The listing builds one solid part. Answer for the finished solid, in the listing's coordinates (mm). A direction names the side the tool comes from. Give positions to 0.01 mm unless a question says otherwise; leave off trailing zeros. Order: outer loops, then holes, each group sorted by start corner. A loop starts at its lowest first (then second) coordinate and runs counter-clockwise, first axis right, second up. Notation, with made-up numbers: (78.25, -32) - (100.25, -32) arc R10 cw to (100.25, -15) - close; hole circle Ø6 at (-38.5, 83). An arc over 180 degrees is marked (long way). Answer as a JSON object with one key per item and string values. Group by question number.
Q1. A cutting plane is placed at A-A, the plane y = 21. Give the vertices of the cut face in (x, z).
Q2. A cutting plane is placed at C-C, the plane y = 12. Give the vertices of the cut face in (x, z).
Q3. A cutting plane is placed at B-B, the plane z = 3.55. Count the separate pieces of the cut face and the enclosed holes in it, and give its area (3 significant figures).
Q4. The mould has two halves that part along X. Classify faces 4 (the face through (-1, 0, 6)), 5 (the face through (70.85, 0, 4)), 6 (the face through (76.592, -21.601, 1.268)): released by +X, released by -X, zero draft, split by the parting line, or undercut.
Q5. Given pin 1 (5 mm diameter, centred on x = 78.5, y = -21, fed in from +Z); pin 2 (1.8 mm diameter, centred on x = 23.5, y = -15, fed in from -Z), each flat-ended and moving along its own axis, determine where each tip first touches the part or whether it passes through.
Q6. Consider line 1 (Y direction, x = 0, z = 2.25) (3 decimals); line 2 (Z direction, x = 71, y = 4.5); line 3 (X direction, y = -0.5, z = 5.05). Determine where each line is inside the solid, lowest interval first.
Q7. For faces 1 (the face through (-79, 0, 2.5)), 2 (the face through (78, 0, 2.5)), 3 (the face through (80.408, 21.601, 1.268)), determine the directions among +Z, -Z, +X, -X, +Y, -Y from which every point of the face is accessible in a straight line to the end or side of a thin tool.
from build123d import *

# Parameters (mm, degrees)
ESQUISSE1_W             = 172
ESQUISSE1_H             = 55
BOSS_EXTRU_1_DEPTH      = 6
ESQUISSE2_W             = 15.15
ESQUISSE2_H             = 55
ENL_V_MAT_EXTRU_1_DEPTH = 3.5
ESQUISSE3_R             = 2
ENL_V_MAT_EXTRU_2_DEPTH = 91.357622811
ESQUISSE4_R             = 1.005
ENL_V_MAT_EXTRU_3_DEPTH = 91.488949602


with BuildPart() as part:
    # Esquisse1 → Boss.-Extru.1 (new body)
    with BuildSketch(Plane.XY):
        Rectangle(ESQUISSE1_W, ESQUISSE1_H)
    extrude(amount=BOSS_EXTRU_1_DEPTH)

    # Esquisse2 → Enlèv. mat.-Extru.1 (cut)
    with BuildSketch(Plane.XY.offset(6)):
        with Locations((-78.425, 0)):
            Rectangle(ESQUISSE2_W, ESQUISSE2_H)
        with Locations((78.425, 0)):
            Rectangle(ESQUISSE2_W, ESQUISSE2_H)
    extrude(amount=-ENL_V_MAT_EXTRU_1_DEPTH, mode=Mode.SUBTRACT)

    # Esquisse3 → Enlèv. mat.-Extru.2 (cut, through all)
    with BuildSketch(Plane.XY.offset(2.5)):
        with Locations(Location((-78.5, 21, 0), (0, 0, 180))):
            Circle(ESQUISSE3_R)
        with Locations((-78.5, -21)):
            Circle(ESQUISSE3_R)
        with Locations(Location((78.5, -21, 0), (0, 0, 180))):
            Circle(ESQUISSE3_R)
        with Locations((78.5, 21)):
            Circle(ESQUISSE3_R)
    extrude(amount=-ENL_V_MAT_EXTRU_2_DEPTH, mode=Mode.SUBTRACT)

    # Esquisse4 → Enlèv. mat.-Extru.3 (cut, through all)
    with BuildSketch(Plane.XY.offset(6)):
        with Locations((-47.35, 15)):
            Circle(ESQUISSE4_R)
        with Locations((-23.5, 15)):
            Circle(ESQUISSE4_R)
        with Locations(Location((23.5, 15, 0), (0, 0, 180))):
            Circle(ESQUISSE4_R)
        with Locations(Location((47.35, 15, 0), (0, 0, 180))):
            Circle(ESQUISSE4_R)
        with Locations((47.35, -15)):
            Circle(ESQUISSE4_R)
        with Locations((23.5, -15)):
            Circle(ESQUISSE4_R)
        with Locations(Location((-23.5, -15, 0), (0, 0, 180))):
            Circle(ESQUISSE4_R)
        with Locations(Location((-47.35, -15, 0), (0, 0, 180))):
            Circle(ESQUISSE4_R)
        with Locations((0, 15)):
            Circle(ESQUISSE4_R)
        with Locations(Location((0, -15, 0), (0, 0, 180))):
            Circle(ESQUISSE4_R)
    extrude(amount=-ENL_V_MAT_EXTRU_3_DEPTH, mode=Mode.SUBTRACT)


solid = part.part
Reply:
{
 "1": {"outline": "(-86, 0) - (-80.5, 0) - (-80.5, 2.5) - (-86, 2.5) - close; (-76.5, 0) - (76.5, 0) - (76.5, 2.5) - (70.85, 2.5) - (70.85, 6) - (-70.85, 6) - (-70.85, 2.5) - (-76.5, 2.5) - close; (80.5, 0) - (86, 0) - (86, 2.5) - (80.5, 2.5) - close"},
 "2": {"outline": "(-86, 0) - (86, 0) - (86, 2.5) - (70.85, 2.5) - (70.85, 6) - (-70.85, 6) - (-70.85, 2.5) - (-86, 2.5) - close"},
 "3": {"separate pieces": "1", "enclosed holes": "10", "area": "7,760 mm^2"},
 "4": {"face 4": "zero draft", "face 5": "released by +X", "face 6": "undercut"},
 "5": {"pin 1": "stops at z = 2.5", "pin 2": "passes through"},
 "6": {"line 1": "y = -27.5 to -16.005, -13.995 to 13.995, 16.005 to 27.5", "line 2": "z = 0 to 2.5", "line 3": "x = -70.85 to 70.85"},
 "7": {"face 1": "+Z, -X, +Y, -Y", "face 2": "+Z, +X, +Y, -Y", "face 3": "+Z, -Z"}
}
